Read the model definition and answer for the solid it produces. Units are mm, in the model's axes. Round coordinates to 2 decimals unless told otherwise and drop trailing zeros. Loops run counter-clockwise (first coordinate to the right, second up) from the corner with the lowest first, then second, coordinate; pieces in that order, holes last. Notation, with made-up numbers: (51, -25.75) - (74, -25.75) arc R21 cw to (74, 2.25) - close; hole circle Ø10 at (59, 61). An arc over 180 degrees is marked (long way). Answer as CSV lines item,"result".
Autodesk Inventor part; units mm, degrees
ref_plane "YZ Plane" through (0, 0, 0) normal (1, 0, 0) x (0, 1, 0)
ref_plane "XZ Plane" through (0, 0, 0) normal (0, 1, 0) x (-1, 0, 0)
ref_plane "XY Plane" through (0, 0, 0) normal (0, 0, 1) x (1, 0, 0)
sketch "Sketch1" plane through (0, 0, 0) normal (1, 0, 0) x (0, 1, 0)
  line L0 (-6.35, 6.35) -> (6.35, 6.35)
  line L1 (6.35, 6.35) -> (6.35, -6.35)
  line L2 (6.35, -6.35) -> (-6.35, -6.35)
  line L3 (-6.35, -6.35) -> (-6.35, 6.35)
  line L4 (-6.35, 6.35) -> (6.35, -6.35) construction
  line L5 (6.35, 6.35) -> (-6.35, -6.35) construction
  point P0 (0, 0)
  dimension "d0" = 12.7
  dimension "d1" = 12.7
extrude "Extrusion1" add sketch "Sketch1" along normal mid plane 365.4
fillet "Fillet1" radius 12.7 3 edges at (0, 6.35, 6.35) (-182.7, 6.35, 0) (182.7, 6.35, 0)
chamfer "Chamfer1" distance 6.35 angle 45 1 edges at (0, -6.35, -6.35)
sketch "Sketch2" plane through (0, 0, 0) normal (0, 0, 1) x (1, 0, 0)
  line L0 (-182.7, -6.35) -> (182.7, -6.35)
  line L1 (170, 6.35) -> (-170, 6.35)
  line L2 (-182.7, -6.35) -> (-182.7, 6.35)
  line L3 (-182.7, 6.35) -> (-170, -6.35)
  line L4 (-182.7, 6.35) -> (-170, 6.35) construction
  point P0 (0, 0)
  dimension "d11" = 45
extrude "Extrusion2" cut sketch "Sketch2" along normal through all both and the other way through all
mirror "Mirror1" about plane through (0, 0, 0) normal (1, 0, 0) of "Extrusion2"
sketch "Sketch3" plane through (0, 0, 0) normal (1, 0, 0) x (0, 1, 0)
  line L0 (-6.35, 6.35) -> (-6.35, 6.35)
  line L1 (-6.35, 0) -> (-6.35, 6.35)
  line L2 (0, -6.35) -> (-6.35, 0)
  line L3 (2.6303, -6.35) -> (0, -6.35)
  line L4 (2.6303, 2.6303) -> (2.6303, -6.35)
  arc A0 (2.6303, 2.6303) -> (-6.35, 6.35) centre (-6.35, -6.35) ccw
  circle A1 centre (0, -6.35) radius 1.5875
  line L5 (6.35, -6.35) -> (2.6303, -6.35)
  point P0 (0, 0)
  dimension "d14" = 3.175
  dimension "d15" = 6.35
extrude "Extrusion3" cut sketch "Sketch3" along normal through all both and the other way through all contours A1 L3 L2 | L2 L3 A1
equation "\"d0\" = facingThickness"
equation "\"d1\" = facingThickness"
equation "\"d7\" = 0.999999 * facingThickness"
equation "\"d4\" = 0.5 * facingThickness"
equation "\"d14\" = 0.25 * facingThickness"
equation "\"d15\" = 0.5 * facingThickness"
equation "\"mppcMountThickness\" = 6.35"
equation "\"facingThickness\" = 12.7"
equation "\"facingGasketThickness\" = 1.5875"
properties part number "frontBackMoulding" material "Wood (Cherry)"
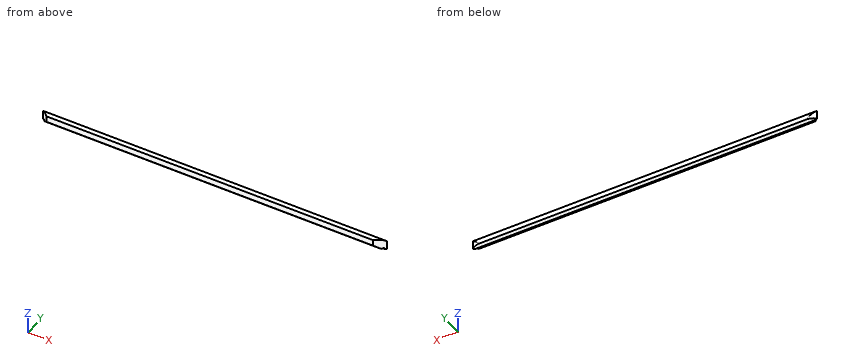
1) Each of these flat-tipped pins is pushed along its axis until it touches: P1, Ø6, axis at x = 94.5, z = -2, coming from the +Y side; P2, Ø1, axis at y = 0, z = -5, coming from the -X side; P3, Ø3, axis at y = -1.5, z = 1.5, coming from the +X side. Where does it stop, or does it pass through?
Entries:
P1,"stops at y = 6.28"
P2,"stops at x = -176.82"
P3,"stops at x = 176.35"
2) A cutting plane is placed at B-B, the plane y = -3.5. Determine the outline of the cut face in (x, z), plus the area to 3 significant figures.
Entries:
outline,"(-172.85, -2.85) - (172.85, -2.85) - (172.85, 6.03) - (-172.85, 6.03) - close"
area,"3,070 mm^2"
3) Find the intervals of material crossed by line 1 (Z direction, x = -66.5, y = 5.25); line 2 (X direction, y = -1.5, z = 0.75); line 3 (X direction, y = -3, z = 3.5), in increasing order.
Entries:
line 1,"z = -6.35 to -1.18"
line 2,"x = -174.85 to 174.85"
line 3,"x = -173.35 to 173.35"
